```python
from build123d import *

# Parameters (mm, degrees)
BOSS_EXTRUDE1_DEPTH    = 25.4
SKETCH2_R              = 2.159
SKETCH2_W              = 12.7
SKETCH2_H              = 1.5875
SKETCH2_W_2            = 1.5875
SKETCH2_H_2            = 12.7
CUT_EXTRUDE1_DEPTH     = 25.4
SKETCH3_W              = 12.7
SKETCH3_H              = 1.5875
SKETCH3_H_2            = 1.5748
CUT_EXTRUDE2_DEPTH     = 12.7
SKETCH4_W              = 1.5875
SKETCH4_H              = 12.7
CUT_EXTRUDE3_DEPTH     = 12.7
F_3DSKETCH1_R          = 19.05
F_3DSKETCH1_R_2        = 11.1125
BOSS_EXTRUDE2_DEPTH    = 11.482870812
CUT_EXTRUDE4_START     = 44.901280605
CUT_EXTRUDE4_OUTLINE_R = 11.1125
CUT_EXTRUDE4_DEPTH     = 11.482870812
SKETCH5_R              = 11.1125
SKETCH5_R_2            = 4.572
BOSS_EXTRUDE3_DEPTH    = 3.81
FILLET1_R              = 5.08
FILLET2_R              = 1.016


# Read off the part's stored shape, not the designer's step: Cut-Extrude4
with BuildPart() as part:
    # Sketch1 → Boss-Extrude1 (new body)
    with BuildSketch(Plane.XY):
        Polygon((88.9, 0), (63.5, 0), (0, -63.5), (0, -88.9), (12.7, -88.9), (12.7, -67.039231637), (67.039231637, -12.7), (88.9, -12.7), align=None)
    extrude(amount=BOSS_EXTRUDE1_DEPTH)

    # Sketch2 → Cut-Extrude1 (cut)
    with BuildSketch(Plane.XY.offset(25.4)):
        with Locations((82.55, -6.3627)):
            Circle(SKETCH2_R)
        with Locations((6.3627, -82.55)):
            Circle(SKETCH2_R)
        with Locations((82.55, -0.79375)):
            Rectangle(SKETCH2_W, SKETCH2_H)
        with Locations((0.79375, -82.55)):
            Rectangle(SKETCH2_W_2, SKETCH2_H_2)
    extrude(amount=-CUT_EXTRUDE1_DEPTH, mode=Mode.SUBTRACT)

    # Sketch3 → Cut-Extrude2 (cut)
    with BuildSketch(Plane.XZ.offset(88.9)):
        with Locations((6.35, 24.60625)):
            Rectangle(SKETCH3_W, SKETCH3_H)
        with Locations((6.35, 0.7874)):
            Rectangle(SKETCH3_W, SKETCH3_H_2)
    extrude(amount=-CUT_EXTRUDE2_DEPTH, mode=Mode.SUBTRACT)

    # Sketch4 → Cut-Extrude3 (cut)
    with BuildSketch(Plane(origin=(88.9, 0, 0), x_dir=(0, 0, -1), z_dir=(1, 0, 0))):
        with Locations((-0.79375, -6.35)):
            Rectangle(SKETCH4_W, SKETCH4_H)
        with Locations((-24.60625, -6.35)):
            Rectangle(SKETCH4_W, SKETCH4_H)
    extrude(amount=-CUT_EXTRUDE3_DEPTH, mode=Mode.SUBTRACT)

    # 3DSketch1 → Boss-Extrude2 (add)
    with BuildSketch(Plane(origin=(67.039231637, -12.7, 0), x_dir=(-0.6713837490692134, -0.6713837490692195, 0.3138275369873187), z_dir=(0.7071067811865508, -0.7071067811865444, 0))):
        with Locations((40.468086778, 0)):
            Circle(F_3DSKETCH1_R)
        with Locations((40.468086778, 0)):
            Circle(F_3DSKETCH1_R_2, mode=Mode.SUBTRACT)
    extrude(amount=-BOSS_EXTRUDE2_DEPTH)

    # Cut-Extrude4 outline → Cut-Extrude4 (cut)
    with BuildSketch(Plane(origin=(0, 0, 0), x_dir=(0.7071067811865438, 0.7071067811865512, 0), z_dir=(0.7071067811865511, -0.7071067811865441, 0)).offset(CUT_EXTRUDE4_START)):
        with Locations((0, 12.7)):
            Circle(CUT_EXTRUDE4_OUTLINE_R)
    extrude(amount=CUT_EXTRUDE4_DEPTH, mode=Mode.SUBTRACT)

    # Sketch5 → Boss-Extrude3 (add)
    with BuildSketch(Plane(origin=(31.75, -31.75, 0), x_dir=(0, 0, 1), z_dir=(-0.7071067811865476, 0.7071067811865475, 0))):
        with Locations(Location((12.7, 0, 0), (0, 0, 270))):
            Circle(SKETCH5_R)
        with Locations(Location((12.7, 0, 0), (0, 0, 270))):
            Circle(SKETCH5_R_2, mode=Mode.SUBTRACT)
    extrude(amount=-BOSS_EXTRUDE3_DEPTH)

    # Fillet1
    fillet1_edges = [part.edges().sort_by_distance(p)[0] for p in [
        (88.9, -1.5875, 12.7),
        (88.9, -12.7, 12.7),
        (63.5, 0, 12.7),
        (67.039231637, -12.7, 12.7),
        (12.7, -67.039231637, 12.7),
        (0, -63.5, 12.7),
        (1.5875, -88.9, 12.69365),
        (12.7, -88.9, 12.69365),
    ]]
    fillet(fillet1_edges, radius=FILLET1_R)

    # Fillet2
    fillet2_edges = [part.edges().sort_by_distance(p)[0] for p in [
        (32.011891712, -47.727339924, 12.7),
    ]]
    fillet(fillet2_edges, radius=FILLET2_R)


solid = part.part
```
Model file for the job. Use its own axes, mm. A direction names the side the tool comes from. Give positions to 0.01 mm unless a question says otherwise; leave off trailing zeros. Write each loop counter-clockwise with the first axis right and the second up, starting at its lowest first coordinate (ties: lowest second). Pieces come first, ordered by that corner, then holes. Notation, with made-up numbers: (-25, 75.5) -> (-8, 75.5) arc R3 cw to (-8, 80.5) -> close; hole circle Ø11 at (56.5, 28). An arc over 180 degrees is marked (long way). Use CSV: the item, a comma, the result in double quotes. Start each with the question number.
1) Drill centre lines: L1, parallel to Z at x = 11.5, y = -53; L2, parallel to Y at x = 30.5, z = 15; L3, parallel to Y at x = 70, z = 17. Where is each one in solid material? Low to high.
2) Cut at A-A on y = -82.55. List the corners of the cut face in (x, z).
3) Cut at D-D on z = 7. Count the separate pieces of the cut face and the enclosed holes in it, plus the area to 3 significant figures.
4) Cut at B-B on x = 82.55. List the corners of the cut face in (y, z).
5) Pin check, flat tips, straight feed: P1, Ø11.5, axis at x = 76, z = 6.5, coming from the -Y side; P2, Ø9, axis at x = 84, y = -7, coming from the -Z side; P3, Ø3.5, axis at x = 81.5, y = -7, coming from the +Z side. Stop position of each tip, or through.
6) Cut at C-C on x = 10.5. List the corners of the cut face in (y, z).
7) Tool access for faces 1 (the flat face through (81.2, -8.5, 23.812)), 2 (the flat face through (80, -1.588, 13)), 3 (the flat face through (12.7, -77, 13)): list every direction of +Z, -Z, +X, -X, +Y, -Y with a clear straight run to the whole face (end or side of a thin tool).
8) Two-plate mould, pull along Y, no slides. Class faces 4 (the cylindrical face through (31.34, -34.816, 16.555)), 5 (the flat face through (11, -59, 25.4)), 6 (the cylindrical face through (87.451, -11.172, 12.856)): released by +Y, released by -Y, zero draft, split by the parting line, or undercut.
Final values:
1,L1,"z = 0 to 25.4"
1,L2,"y = -49.24 to -45.88, -38.39 to -36.09"
1,L3,"y = -12.7 to 0"
2,outline,"(1.59, 1.57) -> (4.2, 1.57) -> (4.2, 23.81) -> (1.59, 23.81) -> close; (8.52, 1.57) -> (12.7, 1.57) -> (12.7, 23.81) -> (8.52, 23.81) -> close"
3,separate pieces,"1"
3,enclosed holes,"2"
3,area,"1,320 mm2"
4,outline,"(-12.7, 1.59) -> (-8.52, 1.59) -> (-8.52, 23.81) -> (-12.7, 23.81) -> close; (-4.2, 1.59) -> (-1.59, 1.59) -> (-1.59, 23.81) -> (-4.2, 23.81) -> close"
5,P1,"stops at y = -12.7"
5,P2,"stops at z = 1.59"
5,P3,"stops at z = 23.81"
6,outline,"(-88, 1.57) -> (-76.2, 1.57) -> (-76.2, 0) -> (-53, 0) -> (-53, 25.4) -> (-76.2, 25.4) -> (-76.2, 23.81) -> (-88, 23.81) -> close"
7,face 1,"+Z, +X, +Y, -Y"
7,face 2,"+Z, -Z, +X, +Y"
7,face 3,"+Z, -Z, +X, -Y"
8,face 4,"undercut"
8,face 5,"zero draft"
8,face 6,"released by -Y"
